CAD build for the part. Positions are in the model's coordinates, mm. A direction names the side the tool comes from. Give positions to 0.01 mm unless a question says otherwise; leave off trailing zeros. Loops run counter-clockwise (first coordinate to the right, second up) from the corner with the lowest first, then second, coordinate; pieces in that order, holes last. Notation, with made-up numbers: (73, 70) -> (128, 70) arc R33 ccw to (128, 105) -> close; hole circle Ø5 at (73.25, 12). An arc over 180 degrees is marked (long way). Write each question's results on one line, items separated by ' | '. Start each with the question number.
```python
from build123d import *

# Parameters (mm, degrees)
F0_W     = 2
F0_H     = 12.7
F0_W_2   = 13.24
F1_DEPTH = 12.7
F3_DEPTH = 12.7
F4_W     = 2.032
F4_H     = 5.08
F5_DEPTH = 12.7
F6_SIZE  = 1.01599
F7_SIZE  = 0.762


# Not quite as in the source:
# - a fillet or chamfer is up to 0.001 mm smaller than in the source, because OpenCascade refuses the exact size


with BuildPart() as f1:
    # F0 (on Top) → F1 (new body)
    with BuildSketch(Plane.XY):
        with Locations((-14.1, 0)):
            Rectangle(F0_W, F0_H)
        with Locations((-21.72, 0)):
            Rectangle(F0_W_2, F0_H)
        with BuildLine():
            ThreePointArc((7.19, 13.1), (11.3690010768, 11.3690010768), (13.1, 7.19))
            Line((13.1, 7.19), (13.1, -7.19))
            ThreePointArc((13.1, -7.19), (11.3690010768, -11.3690010768), (7.19, -13.1))
            Line((7.19, -13.1), (-7.19, -13.1))
            ThreePointArc((-7.19, -13.1), (-11.3690010768, -11.3690010768), (-13.1, -7.19))
            Line((-13.1, -7.19), (-13.1, -6.35))
            Line((-13.1, -6.35), (-15.1, -6.35))
            Line((-15.1, -6.35), (-15.1, -7.19))
            ThreePointArc((-15.1, -7.19), (-12.7832146392, -12.7832146392), (-7.19, -15.1))
            Line((-7.19, -15.1), (7.19, -15.1))
            ThreePointArc((7.19, -15.1), (12.7832146392, -12.7832146392), (15.1, -7.19))
            Line((15.1, -7.19), (15.1, 7.19))
            ThreePointArc((15.1, 7.19), (12.7832146392, 12.7832146392), (7.19, 15.1))
            Line((7.19, 15.1), (-7.19, 15.1))
            ThreePointArc((-7.19, 15.1), (-12.7832146392, 12.7832146392), (-15.1, 7.19))
            Line((-15.1, 7.19), (-15.1, 6.35))
            Line((-15.1, 6.35), (-13.1, 6.35))
            Line((-13.1, 6.35), (-13.1, 7.19))
            ThreePointArc((-13.1, 7.19), (-11.3690010768, 11.3690010768), (-7.19, 13.1))
            Line((-7.19, 13.1), (7.19, 13.1))
        make_face()
    extrude(amount=F1_DEPTH)

    # F2 (on face) → F3 (cut, through all)
    with BuildSketch(Plane.XZ.offset(6.35)):
        with BuildLine():
            ThreePointArc((-28.34, 0), (-26.7817380481, 3.0065509582), (-26.2442648116, 6.35))
            ThreePointArc((-26.2442648116, 6.35), (-26.7817380481, 9.6934490418), (-28.34, 12.7))
            Line((-28.34, 12.7), (-28.34, 0))
        make_face()
    extrude(amount=-F3_DEPTH, mode=Mode.SUBTRACT)

    # F4 (on face) → F5 (cut, through all)
    with BuildSketch(Plane.XY.offset(12.7)):
        with Locations((-21.72, 0)):
            Rectangle(F4_W, F4_H)
    extrude(amount=-F5_DEPTH, mode=Mode.SUBTRACT)

    # F6 (size 1.016 in the source; OpenCascade refuses exactly that, so slightly less here)
    f6_edges = [f1.edges().sort_by_distance(p)[0] for p in [
        (-22.736, -2.54, 6.35),
        (-20.704, -2.54, 6.35),
        (-20.704, 2.54, 6.35),
        (-22.736, 2.54, 6.35),
    ]]
    chamfer(f6_edges, length=F6_SIZE)

    # F7
    f7_edges = [f1.edges().sort_by_distance(p)[0] for p in [
        (-11.369001, -11.369001, 12.7),
        (0, -13.1, 12.7),
        (-13.1, 0, 12.7),
        (-11.369001, 11.369001, 12.7),
        (0, 13.1, 12.7),
        (11.369001, 11.369001, 12.7),
        (13.1, 0, 12.7),
        (11.369001, -11.369001, 12.7),
    ]]
    chamfer(f7_edges, length=F7_SIZE)


solid = f1.part
```
Q1. Drop flat-ended pins along their axis: pin 1 (3 mm diameter, centred on x = -21.5, y = -8, fed in from -Z); pin 2 (6.5 mm diameter, centred on x = -23, z = 5.5, fed in from +Y); pin 3 (1.5 mm diameter, centred on y = -8, z = 6.5, fed in from -X); pin 4 (1 mm diameter, centred on y = -9.5, z = 10, fed in from -X). Give the stop position or say it passes through.
Q2. Saw through at A-A, the plane y = 3. List the corners of the cut face in (x, z), then the cut area to 3 significant figures.
Q3. Saw through at D-D, the plane z = 11.25. Give the number of separate pieces and of enclosed holes in the cut face, then the cut area to 3 significant figures.
Q4. Saw through at C-C, the plane x = -6.5. List the corners of the cut face in (y, z).
Q5. Mould opens along Y. For faces 1 (the face through (-22.24, 2.02, 6.44)), 2 (the face through (15.1, 0, 6)), 3 (the face through (0, -15.1, 6)), 4 (the face through (0, 15.1, 6)) say: pulls with the +Y half, pulls with the -Y half, needs draft (parallel to the pull), parting line crosses it, or undercut.
Q6. Which spindle directions (+Z, -Z, +X, -X, +Y, -Y) get a long thin tool onto all of the face, cutting with end or side? Do faces 5 (the face through (11.415, 11.509, 12.07)), 6 (the face through (-13.1, 0, 6)), 7 (the face through (12.721, -12.844, 6.261)). Say none if no direction does.
Q7. Wall check: L1, parallel to Y at x = 1, z = 10.5; L2, parallel to X at y = 10, z = 6.75; L3, parallel to X at y = 4, z = 10.5. Give the ranges that are in metal, low to high.
Q8. Saw through at B-B, the plane y = -0.5. List the corners of the cut face in (x, z), then the cut area to 3 significant figures.
Answer block:
1) pin 1: passes through | pin 2: stops at y = 6.35 | pin 3: stops at x = -15.1 | pin 4: stops at x = -14.89
2) outline: (-28.34, 0) -> (-13.1, 0) -> (-13.1, 11.94) -> (-13.86, 12.7) -> (-28.34, 12.7) arc R10.67 cw to start; (13.1, 0) -> (15.1, 0) -> (15.1, 12.7) -> (13.86, 12.7) -> (13.1, 11.94) -> close | area: 200 mm2
3) separate pieces: 1 | enclosed holes: 2 | area: 350 mm2
4) outline: (-15.1, 0) -> (-13.1, 0) -> (-13.1, 11.94) -> (-13.86, 12.7) -> (-15.1, 12.7) -> close; (13.1, 0) -> (15.1, 0) -> (15.1, 12.7) -> (13.86, 12.7) -> (13.1, 11.94) -> close
5) face 1: undercut | face 2: needs draft | face 3: pulls with the -Y half | face 4: pulls with the +Y half
6) face 5: +Z | face 6: +Z, -Z | face 7: +Z, -Z, +X, -Y
7) L1: y = -15.1 to -13.1, 13.1 to 15.1 | L2: x = -14.58 to -12.39, 12.39 to 14.58 | L3: x = -27.08 to -13.1, 13.1 to 15.1
8) outline: (-28.34, 0) -> (-22.74, 0) -> (-22.74, 12.7) -> (-28.34, 12.7) arc R10.67 cw to start; (-20.7, 0) -> (-13.1, 0) -> (-13.1, 11.94) -> (-13.86, 12.7) -> (-20.7, 12.7) -> close; (13.1, 0) -> (15.1, 0) -> (15.1, 12.7) -> (13.86, 12.7) -> (13.1, 11.94) -> close | area: 174 mm2
